Input: part model. Units: mm. Frame: model coordinates. Face numbers are marked on the shaded views. A direction names the side the tool comes from. Give positions to 0.01 mm unless a question says otherwise; leave off trailing zeros. Loops run counter-clockwise (first coordinate to the right, second up) from the corner with the lowest first, then second, coordinate; pieces in that order, holes last. Notation, with made-up numbers: (-21.5, 86) - (0.5, 86) arc R23 ccw to (0.5, 99) - close; hole circle Ø10 at (40, -23.75). An arc over 180 degrees is marked (long way). Answer as a JSON object with one key per item and string values. Group by question number.
(1) Mould query, pull axis Y, two halves, no side actions, for the marked faces 1, 2 and 3. Classes: +Y half, -Y half, draft (parallel to the pull), parting line (faces both ways), or undercut.
(2) Section query A-A (y = 0). Return loops of the section in (x, z).
(3) Pin query (flat end, axial travel): P1, Ø6, axis at x = 20.5, y = 14, coming from the +Z side; P2, Ø2, axis at y = -25, z = 12.5, coming from the -X side; P3, Ø12, axis at y = -25, z = 19, coming from the +X side. Return the tip coordinate at first contact, or that it passes through.
(4) Section query C-C (x = 0). Return loops of the section in (y, z).
(5) Section query D-D (y = 22.5). Return loops of the section in (x, z).
(6) Material intervals for L1, parallel to X at y = -24, z = 10.5; L2, parallel to X at y = -20.5, z = 6.5; L3, parallel to Y at x = 9.5, z = 12.25, sorted ascending.
(7) Section query B-B (z = 10). Return loops of the section in (x, y), plus the area to 3 significant figures.
(8) Access query for the marked faces 4, 5 and 6. Directions: +Z, -Z, +X, -X, +Y, -Y. A direction counts if a zero-diameter tool reaches every point of the face in a straight line with its end or side. Return the directions, or none.
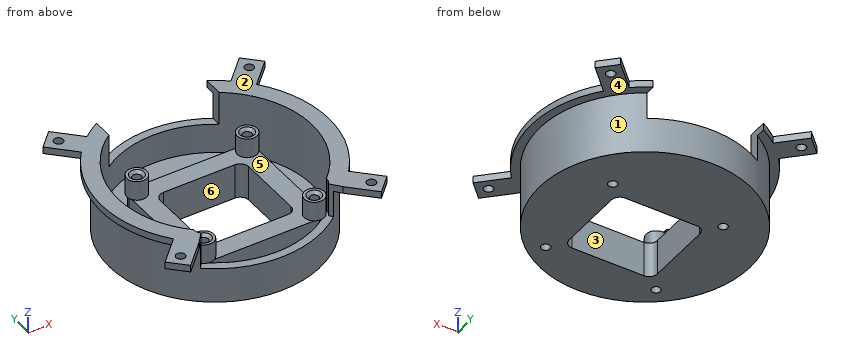
```python
from build123d import *

# Parameters (mm, degrees)
BOSS_EXTRUDE1_DEPTH     = 10.8
CUT_EXTRUDE1_DEPTH      = 63.509359299
CUT_EXTRUDE1_DEPTH_BACK = 63.509359299
SKETCH14_W              = 32
SKETCH14_H              = 30
CUT_EXTRUDE3_DEPTH      = 60.51688836
FILLET1_R               = 3
SKETCH16_R              = 1.6
CUT_EXTRUDE2_DEPTH      = 60.51688836
CUT_EXTRUDE4_DEPTH      = 75.590213715
BOSS_EXTRUDE3_START     = -2.5
SKETCH22_R              = 1.65
BOSS_EXTRUDE3_DEPTH     = 2.5
BOSS_EXTRUDE4_START     = 7.1
SKETCH24_R              = 3.6
SKETCH24_R_2            = 1.6
BOSS_EXTRUDE4_DEPTH     = 7.1
CHAMFER1_SIZE           = 1
CUT_EXTRUDE5_START      = -12.2
CUT_EXTRUDE5_DEPTH      = 12.2


# Read off the part's stored shape, not the designer's step: Cut-Extrude5
with BuildPart() as part:
    # Sketch6 → Revolve1 (revolve)
    with BuildSketch(Plane(origin=(0, 0, 0), x_dir=(0, 0, -1), z_dir=(1, 0, 0)), mode=Mode.PRIVATE) as revolve1_sk:
        Polygon((-2, 25.4), (-2, 35.1), (-25, 35.1), (-25, 37.95), (-25, 41.1), (-22.5, 41.1), (-22.5, 38.1), (0, 38.1), (0, 25.4), (0, 0), (-2, 0), align=None)
    revolve(revolve1_sk.sketch.rotate(Axis((0, 0, 0), (0, 0, 1)), 90), axis=Axis((0, 0, 0), (0, 0, 1)))

    # Sketch15 → Boss-Extrude1 (add)
    with BuildSketch(Plane.XY.offset(2)):
        with BuildLine():
            Line((-20, 15.904297927), (20, 15.904297927))
            ThreePointArc((20, 15.904297927), (22.121320344, 15.02561827), (23, 12.904297927))
            Line((23, 12.904297927), (23, -24.995702073))
            ThreePointArc((23, -24.995702073), (22.121320344, -27.117022417), (20, -27.995702073))
            Line((20, -27.995702073), (-20, -27.995702073))
            ThreePointArc((-20, -27.995702073), (-22.121320344, -27.117022417), (-23, -24.995702073))
            Line((-23, -24.995702073), (-23, 12.904297927))
            ThreePointArc((-23, 12.904297927), (-22.121320344, 15.02561827), (-20, 15.904297927))
        make_face()
    extrude(amount=BOSS_EXTRUDE1_DEPTH)

    # Sketch14 → Cut-Extrude1 (cut, two sides: drawn at the far end of the back side and taken through both)
    with BuildSketch(Plane.XY.offset(2).offset(-CUT_EXTRUDE1_DEPTH_BACK)):
        with Locations((-0.00164643, -5.995702073)):
            Rectangle(SKETCH14_W, SKETCH14_H)
    extrude(amount=CUT_EXTRUDE1_DEPTH + CUT_EXTRUDE1_DEPTH_BACK, mode=Mode.SUBTRACT)

    # Sketch18 → Cut-Extrude3 (cut, through all)
    with BuildSketch(Plane.XY.offset(12.8)):
        with BuildLine():
            Line((19.99835357, -24.995702073), (23.99835357, -24.995702073))
            Line((23.99835357, -24.995702073), (23.99835357, -25.995702073))
            ThreePointArc((23.99835357, -25.995702073), (23.119673914, -28.117022417), (20.99835357, -28.995702073))
            Line((20.99835357, -28.995702073), (19.99835357, -28.995702073))
            Line((19.99835357, -28.995702073), (19.99835357, -24.995702073))
        make_face()
        with BuildLine():
            Line((-20.00164643, -24.995702073), (-24.00164643, -24.995702073))
            Line((-24.00164643, -24.995702073), (-24.00164643, -25.995702073))
            ThreePointArc((-24.00164643, -25.995702073), (-23.122966774, -28.117022417), (-21.00164643, -28.995702073))
            Line((-21.00164643, -28.995702073), (-20.00164643, -28.995702073))
            Line((-20.00164643, -28.995702073), (-20.00164643, -24.995702073))
        make_face()
    extrude(amount=CUT_EXTRUDE3_DEPTH, mode=Mode.SUBTRACT)

    # Fillet1
    fillet1_edges = [part.edges().sort_by_distance(p)[0] for p in [
        (-16.00164643, 9.004297927, 6.4),
        (-16.00164643, -20.995702073, 6.4),
        (15.99835357, -20.995702073, 6.4),
        (15.99835357, 9.004297927, 6.4),
    ]]
    fillet(fillet1_edges, radius=FILLET1_R)

    # Sketch16 → Cut-Extrude2 (cut, through all)
    with BuildSketch(Plane.XY.offset(12.8)):
        with Locations((-20.00164643, 13.004297927)):
            Circle(SKETCH16_R)
        with Locations((-20.00164643, -24.995702073)):
            Circle(SKETCH16_R)
        with Locations((19.99835357, -24.995702073)):
            Circle(SKETCH16_R)
        with Locations((19.99835357, 13.004297927)):
            Circle(SKETCH16_R)
    extrude(amount=-CUT_EXTRUDE2_DEPTH, mode=Mode.SUBTRACT)

    # Sketch20 → Cut-Extrude4 (cut, through all)
    with BuildSketch(Plane(origin=(0, 15.904297927, 0), x_dir=(1, 0, 0), z_dir=(0, 1, 0))):
        Polygon((20, -12.8), (-20, -12.8), (-20, -25), (19.99835357, -25), align=None)
    extrude(amount=CUT_EXTRUDE4_DEPTH, mode=Mode.SUBTRACT)

    # Sketch22 → Boss-Extrude3 (add)
    # profile 1 of 2: a face of its own
    with BuildSketch(Plane.XY.offset(25).offset(BOSS_EXTRUDE3_START)):
        with BuildLine():
            Line((-40.237833378, 34.580979128), (-31.752552003, 26.095697754))
            ThreePointArc((-31.752552003, 26.095697754), (-29.062088707, 29.062088707), (-26.095697754, 31.752552003))
            Line((-26.095697754, 31.752552003), (-34.580979128, 40.237833378))
            Line((-34.580979128, 40.237833378), (-40.237833378, 34.580979128))
        make_face()
        with Locations((-34.580979128, 34.580979128)):
            Circle(SKETCH22_R, mode=Mode.SUBTRACT)
    # profile 2 of 2: a face of its own
    with BuildSketch(Plane.XY.offset(25).offset(BOSS_EXTRUDE3_START)):
        with BuildLine():
            ThreePointArc((26.095697754, 31.752552003), (29.062088707, 29.062088707), (31.752552003, 26.095697754))
            Line((31.752552003, 26.095697754), (40.237833378, 34.580979128))
            Line((40.237833378, 34.580979128), (34.580979128, 40.237833378))
            Line((34.580979128, 40.237833378), (26.095697754, 31.752552003))
        make_face()
        with Locations((34.580979128, 34.580979128)):
            Circle(SKETCH22_R, mode=Mode.SUBTRACT)
    boss_extrude3 = extrude(amount=BOSS_EXTRUDE3_DEPTH)

    # Sketch24 → Boss-Extrude4 (add)
    # profile 1 of 4: a face of its own
    with BuildSketch(Plane.XY.offset(12.8).offset(BOSS_EXTRUDE4_START)):
        with Locations(Location((-20.00164643, 13.004297927, 0), (0, 0, 213.6046846))):
            Circle(SKETCH24_R)
        with Locations((-20.00164643, 13.004297927)):
            Circle(SKETCH24_R_2, mode=Mode.SUBTRACT)
    # profile 2 of 4: a face of its own
    with BuildSketch(Plane.XY.offset(12.8).offset(BOSS_EXTRUDE4_START)):
        with Locations(Location((19.99835357, 13.004297927, 0), (0, 0, 126.336057515))):
            Circle(SKETCH24_R)
        with Locations((19.99835357, 13.004297927)):
            Circle(SKETCH24_R_2, mode=Mode.SUBTRACT)
    # profile 3 of 4: a face of its own
    with BuildSketch(Plane.XY.offset(12.8).offset(BOSS_EXTRUDE4_START)):
        with Locations(Location((-20.00164643, -24.995702073, 0), (0, 0, 198.741091164))):
            Circle(SKETCH24_R)
        with Locations((-20.00164643, -24.995702073)):
            Circle(SKETCH24_R_2, mode=Mode.SUBTRACT)
    # profile 4 of 4: a face of its own
    with BuildSketch(Plane.XY.offset(12.8).offset(BOSS_EXTRUDE4_START)):
        with Locations(Location((19.99835357, -24.995702073, 0), (0, 0, 236.442690237))):
            Circle(SKETCH24_R)
        with Locations((19.99835357, -24.995702073)):
            Circle(SKETCH24_R_2, mode=Mode.SUBTRACT)
    extrude(amount=-BOSS_EXTRUDE4_DEPTH)

    # Chamfer1
    chamfer1_edges = [part.edges().sort_by_distance(p)[0] for p in [
        (-21.60164643, 13.004297927, 19.9),
        (18.39835357, 13.004297927, 19.9),
        (-21.60164643, -24.995702073, 19.9),
        (18.39835357, -24.995702073, 19.9),
    ]]
    chamfer(chamfer1_edges, length=CHAMFER1_SIZE)

    # Mirror1: Boss-Extrude3 across plane
    add(boss_extrude3.mirror(Plane.ZX))

    # Cut-Extrude5 outline → Cut-Extrude5 (cut)
    with BuildSketch(Plane.XY.offset(25).offset(CUT_EXTRUDE5_START)):
        with BuildLine():
            ThreePointArc((-26.095697754, -31.752552003), (0, -41.1), (26.095697754, -31.752552003))
            Line((26.095697754, -31.752552003), (23.119673914, -28.117022417))
            ThreePointArc((23.119673914, -28.117022417), (22.146403867, -28.767340671), (20.99835357, -28.995702073))
            Line((20.99835357, -28.995702073), (19.99835357, -28.995702073))
            Line((19.99835357, -28.995702073), (19.99835357, -28.845725064))
            ThreePointArc((19.99835357, -28.845725064), (-0.002003485, -35.099999943), (-20.00164643, -28.843441891))
            Line((-20.00164643, -28.843441891), (-20.00164643, -28.995702073))
            Line((-20.00164643, -28.995702073), (-21.00164643, -28.995702073))
            ThreePointArc((-21.00164643, -28.995702073), (-22.144276194, -28.769579725), (-23.11465654, -28.125300222))
            Line((-23.11465654, -28.125300222), (-26.095697754, -31.752552003))
        make_face()
    extrude(amount=CUT_EXTRUDE5_DEPTH, mode=Mode.SUBTRACT)


solid = part.part
```
Recorded:
{
 "1": {"face 1": "parting line", "face 2": "draft", "face 3": "undercut"},
 "2": {"outline": "(-41.1, 22.5) - (-38.1, 22.5) - (-38.1, 0) - (-16, 0) - (-16, 12.8) - (-23, 12.8) - (-23, 2) - (-35.1, 2) - (-35.1, 25) - (-41.1, 25) - close; (16, 0) - (38.1, 0) - (38.1, 22.5) - (41.1, 22.5) - (41.1, 25) - (35.1, 25) - (35.1, 2) - (23, 2) - (23, 12.8) - (16, 12.8) - close"},
 "3": {"P1": "stops at z = 19.9", "P2": "stops at x = -29.59", "P3": "stops at x = 35.83"},
 "4": {"outline": "(-38.1, 0) - (-21, 0) - (-21, 12.8) - (-28, 12.8) - (-28, 2) - (-35.1, 2) - (-35.1, 12.8) - (-38.1, 12.8) - close; (9, 0) - (38.1, 0) - (38.1, 12.8) - (35.1, 12.8) - (35.1, 2) - (15.9, 2) - (15.9, 12.8) - (9, 12.8) - close"},
 "5": {"outline": "(-34.39, 22.5) - (-30.75, 22.5) - (-30.75, 0) - (30.75, 0) - (30.75, 22.5) - (34.39, 22.5) - (34.39, 25) - (26.94, 25) - (26.94, 2) - (-26.94, 2) - (-26.94, 25) - (-34.39, 25) - close"},
 "6": {"L1": "x = -29.59 to -25.61, -23 to -21.25, -18.75 to 18.75, 21.25 to 23, 25.61 to 29.59", "L2": "x = -32.11 to -28.49, -23 to -14.65, 14.65 to 23, 28.49 to 32.11", "L3": "y = -36.9 to -33.79, -28 to -21, 9 to 15.9, 33.79 to 36.9"},
 "7": {"outline": "circle Ø76.2 at (0, 0); (-23, -25) arc R3 ccw to (-20, -28) - (20, -28) arc R3 ccw to (23, -25) - (23, 12.9) arc R3 ccw to (20, 15.9) - (-20, 15.9) arc R3 ccw to (-23, 12.9) - close; hole circle Ø70.2 at (0, 0); hole circle Ø3.2 at (-20, -25); hole circle Ø3.2 at (-20, 13); hole (-16, -18) arc R3 ccw to (-13, -21) - (13, -21) arc R3 ccw to (16, -18) - (16, 6) arc R3 ccw to (13, 9) - (-13, 9) arc R3 ccw to (-16, 6) - close; hole circle Ø3.2 at (20, -25); hole circle Ø3.2 at (20, 13)", "area": "1,720 mm^2"},
 "8": {"face 4": "-Z, +X", "face 5": "+Z", "face 6": "+Z, -Z"}
}
